Model file for the job. Use its own axes, mm. A direction names the side the tool comes from. Round coordinates to 2 decimals unless told otherwise and drop trailing zeros. Order: outer loops, then holes, each group sorted by start corner. A loop starts at its lowest first (then second) coordinate and runs counter-clockwise, first axis right, second up. Notation, with made-up numbers: (-19.5, 24) -> (24.5, 24) arc R10 ccw to (24.5, 34) -> close; hole circle Ø1 at (-29, 40.25). An arc over 180 degrees is marked (long way). Answer as CSV lines item,"result".
```python
from build123d import *

# Parameters (mm, degrees)
SKETCH2_R               = 5
BOSS_EXTRUDE1_DEPTH     = 19.939
CUT_EXTRUDE1_DEPTH      = 141.037239765
CUT_EXTRUDE1_DEPTH_BACK = 141.037239765
SKETCH3_W               = 25.878
SKETCH3_H               = 67.31
FILLET1_R               = 4


with BuildPart() as part:
    # Sketch2 → Boss-Extrude1 (new, symmetric)
    with BuildSketch(Plane.YZ):
        with BuildLine():
            Line((-33.02, 0), (33.02, 0))
            Line((33.02, 0), (33.02, 101.6))
            ThreePointArc((33.02, 101.6), (21.345667043, 106.435667043), (16.51, 118.11))
            ThreePointArc((16.51, 118.11), (0, 134.62), (-16.51, 118.11))
            ThreePointArc((-16.51, 118.11), (-21.345667043, 106.435667043), (-33.02, 101.6))
            Line((-33.02, 101.6), (-33.02, 0))
        make_face()
        with Locations(Location((0, 118.11, 0), (0, 0, 270))):
            Circle(SKETCH2_R, mode=Mode.SUBTRACT)
    extrude(amount=BOSS_EXTRUDE1_DEPTH, both=True)

    # Sketch3 → Cut-Extrude1 (cut, two sides: drawn at the far end of the back side and taken through both)
    with BuildSketch(Plane(origin=(0, 0, 0), x_dir=(-1, 0, 0), z_dir=(0, 1, 0)).offset(-CUT_EXTRUDE1_DEPTH_BACK)):
        with Locations((0, 100.965)):
            Rectangle(SKETCH3_W, SKETCH3_H)
    extrude(amount=CUT_EXTRUDE1_DEPTH + CUT_EXTRUDE1_DEPTH_BACK, mode=Mode.SUBTRACT)

    # Fillet1
    fillet1_edges = [part.edges().sort_by_distance(p)[0] for p in [
        (12.939, 33.02, 84.455),
        (-12.939, -33.02, 84.455),
        (0, -33.02, 67.31),
        (-12.939, 33.02, 84.455),
        (12.939, -33.02, 84.455),
        (12.939, 0, 67.31),
        (-12.939, 0, 67.31),
        (0, 33.02, 67.31),
    ]]
    fillet(fillet1_edges, radius=FILLET1_R)


solid = part.part
```
Q1. Saw through at B-B (z = 99.5). Write the cut outline in (x, y), plus the area to 3 significant figures.
Checks:
outline,"(-19.94, -33.02) -> (-16.94, -33.02) arc R4 ccw to (-12.94, -29.02) -> (-12.94, 29.02) arc R4 ccw to (-16.94, 33.02) -> (-19.94, 33.02) -> close; (12.94, -29.02) arc R4 ccw to (16.94, -33.02) -> (19.94, -33.02) -> (19.94, 33.02) -> (16.94, 33.02) arc R4 ccw to (12.94, 29.02) -> close"
area,"911 mm²"
Q2. Tool access for faces 4 (the cylindrical face through (14.08, 31.82, 86.49)), 5 (the cylindrical face through (-11.736, 0.406, 68.451)), 6 (the cylindrical face through (14.14, -31.88, 86.92)): list every direction of +Z, -Z, +X, -X, +Y, -Y with a clear straight run to the whole face (end or side of a thin tool).
Checks:
face 4,"+Z, +Y"
face 5,"+Z, +Y, -Y"
face 6,"+Z, -Y"
Q3. Flat gauge pins, fed straight in: pin 1 (2 mm diameter, centred on x = 14.5, y = -7, fed in from +Z); pin 2 (10 mm diameter, centred on x = 8.5, z = 99.5, fed in from +Y); pin 3 (12 mm diameter, centred on x = 10.5, y = 12.5, fed in from +Z); pin 4 (16 mm diameter, centred on y = 0, z = 118.11, fed in from -X). Where does each tip first touch, or does it go through?
Checks:
pin 1,"z = 133.49"
pin 2,"y = 31.06"
pin 3,"z = 133.05"
pin 4,"x = -19.94"
Q4. Saw through at D-D (y = -12). Write the cut outline in (x, z), plus the area to 3 significant figures.
Checks:
outline,"(-19.94, 0) -> (19.94, 0) -> (19.94, 129.45) -> (12.94, 129.45) -> (12.94, 71.31) arc R4 cw to (8.94, 67.31) -> (-8.94, 67.31) arc R4 cw to (-12.94, 71.31) -> (-12.94, 129.45) -> (-19.94, 129.45) -> close"
area,"3,560 mm²"
Q5. Wall check: L1, parallel to X at y = -2.5, z = 111; L2, parallel to Z at x = 14.5, y = 0; L3, parallel to Y at x = -18, z = 118. Give the ranges that are in metal, low to high. Write a range as [from, to].
Checks:
L1,"[-19.94, -12.94], [12.94, 19.94]"
L2,"[0, 113.11], [123.11, 134.62]"
L3,"[-16.51, -5], [5, 16.51]"
Q6. Saw through at C-C (x = 4). Write the cut outline in (y, z).
Checks:
outline,"(-33.02, 0) -> (33.02, 0) -> (33.02, 63.31) arc R4 ccw to (29.02, 67.31) -> (-29.02, 67.31) arc R4 ccw to (-33.02, 63.31) -> close"
Q7. Saw through at A-A (y = 0). Write the cut outline in (x, z).
Checks:
outline,"(-19.94, 0) -> (19.94, 0) -> (19.94, 113.11) -> (12.94, 113.11) -> (12.94, 71.31) arc R4 cw to (8.94, 67.31) -> (-8.94, 67.31) arc R4 cw to (-12.94, 71.31) -> (-12.94, 113.11) -> (-19.94, 113.11) -> close; (-19.94, 123.11) -> (-12.94, 123.11) -> (-12.94, 134.62) -> (-19.94, 134.62) -> close; (12.94, 123.11) -> (19.94, 123.11) -> (19.94, 134.62) -> (12.94, 134.62) -> close"
Q8. Mould opens along Z. For faces 1 (the flat face through (-12.939, 0, 95)), 2 (the cylindrical face through (16.39, 0.22, 123.105)), 3 (the flat face through (0, 0, 0)) say: +Z half, -Z half, draft (parallel to the pull), parting line (faces both ways), or undercut.
Checks:
face 1,"draft"
face 2,"undercut"
face 3,"-Z half"
